Part print with two shaded views. Sizes in mm from the minimum x, y, z corner. A direction names the side the tool comes from. Round coordinates to 2 decimals unless told otherwise and drop trailing zeros. Loops run counter-clockwise (first coordinate to the right, second up) from the corner with the lowest first, then second, coordinate; pieces in that order, holes last. Notation, with made-up numbers: (63, -20.5) -> (92, -20.5) arc R16 ccw to (92, -5.5) -> close; hole circle Ø10 at (35.25, 75.5). An arc over 180 degrees is marked (long way). Use a Markdown table: item, result. Add a question column.
Item 1: Probe line 1 (Z direction, x = 4.75, y = 8); line 2 (Y direction, x = 1.25, z = 8); line 3 (Y direction, x = 0.5, z = 8.5) (1 decimal). List the from-to ranges inside material, lowest first. Write a range as [from, to].
Item 2: Cut at B-B, the plane y = 23. List the corners of the cut face in (x, z).
Item 3: Which spindle directions (+Z, -Z, +X, -X, +Y, -Y) get a long thin tool onto all of the face, cutting with end or side? Do the marked faces 1, 2 and 3. Say none if no direction does.
Item 4: Cut at A-A, the plane x = 4.7. List the corners of the cut face in (y, z), plus the area to 3 significant figures.
Item 5: Flat gauge pins, fed straight in: pin 1 (4 mm diameter, centred on x = 2.5, y = 12.5, fed in from +Z) (1 decimal); pin 2 (0.6 mm diameter, centred on y = 23, z = 0.5, fed in from -X); pin 3 (4 mm diameter, centred on x = 5, y = 15, fed in from -Z). Where does each tip first touch, or does it go through?
Item 6: Cut at C-C, the plane y = 27. List the corners of the cut face in (x, z).
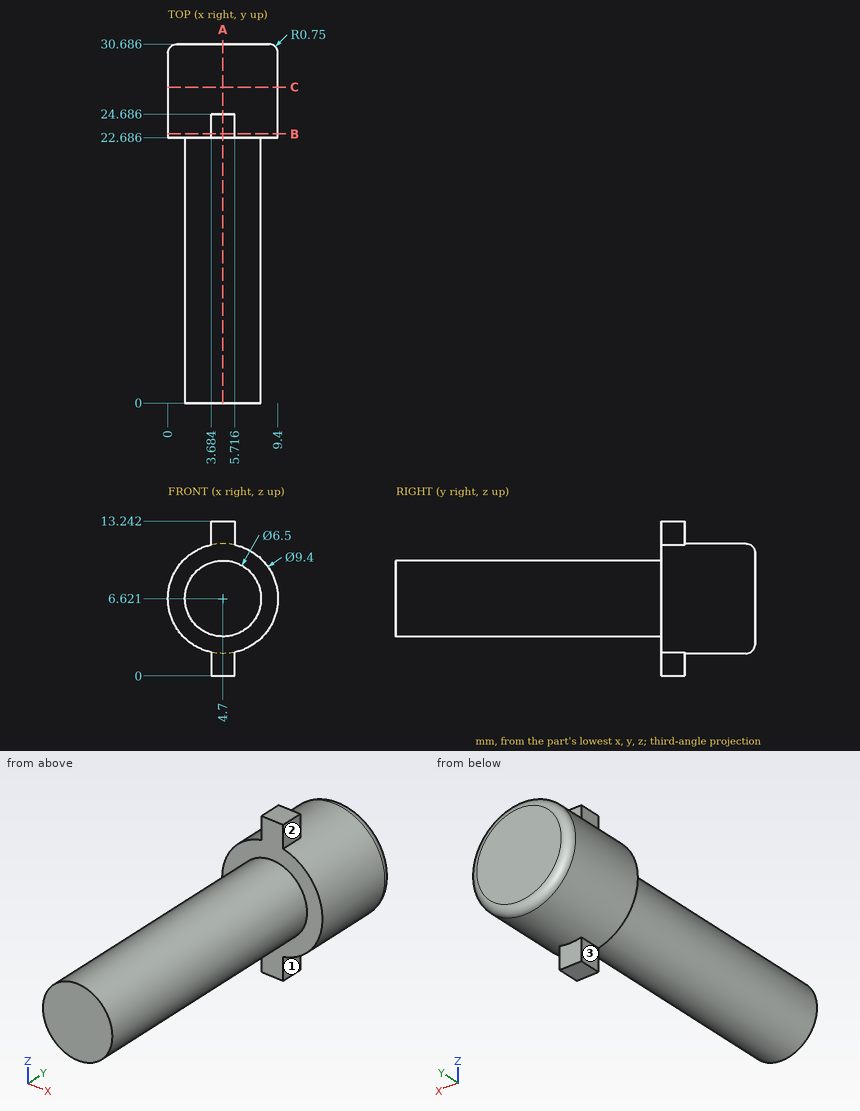
A:
| question | item | result |
|---|---|---|
| 1 | line 1 | z = [3.37, 9.87] |
| 1 | line 2 | y = [22.69, 30.69] |
| 1 | line 3 | y = [22.7, 30.3] |
| 2 | outline | (3.68, 0) -> (5.72, 0) -> (5.72, 2.03) arc R4.7 ccw to (5.72, 11.21) -> (5.72, 13.24) -> (3.68, 13.24) -> (3.68, 11.21) arc R4.7 ccw to (3.68, 2.03) -> close |
| 3 | face 1 | -Z, +X, +Y, -Y |
| 3 | face 2 | +Z, +X, +Y, -Y |
| 3 | face 3 | -Z, -X, +Y, -Y |
| 4 | outline | (0, 3.37) -> (22.69, 3.37) -> (22.69, 0) -> (24.69, 0) -> (24.69, 1.92) -> (29.94, 1.92) arc R0.75 ccw to (30.69, 2.67) -> (30.69, 10.57) arc R0.75 ccw to (29.94, 11.32) -> (24.69, 11.32) -> (24.69, 13.24) -> (22.69, 13.24) -> (22.69, 9.87) -> (0, 9.87) -> close |
| 4 | area | 230 mm^2 |
| 5 | pin 1 | stops at z = 9.9 |
| 5 | pin 2 | stops at x = 3.68 |
| 5 | pin 3 | stops at z = 3.37 |
| 6 | outline | circle Ø9.4 at (4.7, 6.62) |
